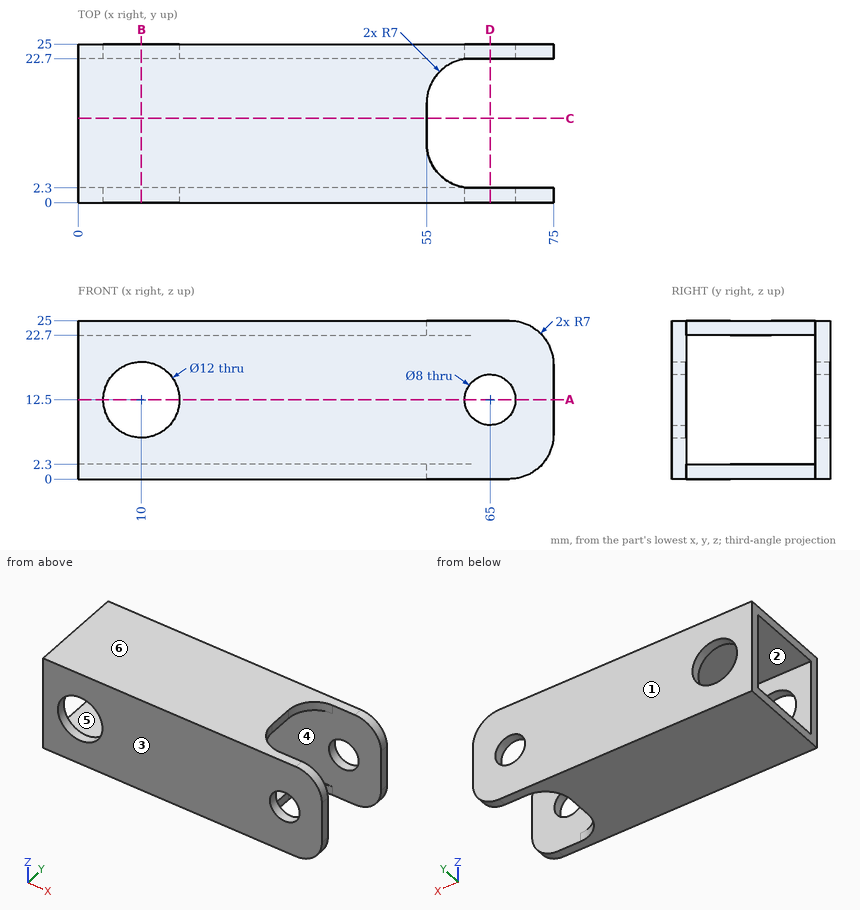
Design review of the part shown in the three views and the two pictorial views. Dimensions are in mm from the part's minimum x, y and z. A direction names the side the tool comes from. Coordinates: 2 decimals unless noted, no trailing zeros. Loops run counter-clockwise (first coordinate to the right, second up) from the corner with the lowest first, then second, coordinate; pieces in that order, holes last.
Q1. We need section B-B on x = 10. State the section outline as (y, z) points, and give its area (3 significant figures).
Reported:
outline: (0, 0) - (25, 0) - (25, 6.5) - (22.7, 6.5) - (22.7, 2.3) - (2.3, 2.3) - (2.3, 6.5) - (0, 6.5) - close; (0, 18.5) - (2.3, 18.5) - (2.3, 22.7) - (22.7, 22.7) - (22.7, 18.5) - (25, 18.5) - (25, 25) - (0, 25) - close
area: 154 mm2
Q2. We need section C-C on y = 13.25. State the section outline as (x, z) points.
Reported:
outline: (0, 0) - (55, 0) - (55, 2.3) - (0, 2.3) - close; (0, 22.7) - (55, 22.7) - (55, 25) - (0, 25) - close
Q3. To check wall thickness, follow line 1 (X direction, y = 23.4, z = 12.5); line 2 (Z direction, x = 10, y = 1.7); line 3 (Z direction, x = 37.5, y = 13). State the ranges of each line that lie inside material, in increasing order.
Reported:
line 1: x = 0 to 4, 16 to 61, 69 to 75
line 2: z = 0 to 6.5, 18.5 to 25
line 3: z = 0 to 2.3, 22.7 to 25
Q4. The part is to be moulded in two halves that separate along Y. For the marked faces 1, 2, 3 and 4, say which applies: +Y half, -Y half, draft (parallel to the pull), parting line (faces both ways), or undercut.
Reported:
face 1: +Y half
face 2: undercut
face 3: -Y half
face 4: undercut
Q5. For pin 1 (10 mm diameter, centred on y = 10, z = 18.5, fed in from +X); pin 2 (1.8 mm diameter, centred on y = 11.5, z = 1, fed in from +X), all flat-tipped, find the tip position at first contact; note any pin that passes through.
Reported:
pin 1: stops at x = 55.3
pin 2: stops at x = 55
Q6. We need section D-D on x = 65. State the section outline as (y, z) points.
Reported:
outline: (0, 0) - (2.3, 0) - (2.3, 8.5) - (0, 8.5) - close; (0, 16.5) - (2.3, 16.5) - (2.3, 25) - (0, 25) - close; (22.7, 0) - (25, 0) - (25, 8.5) - (22.7, 8.5) - close; (22.7, 16.5) - (25, 16.5) - (25, 25) - (22.7, 25) - close
Q7. Tool access review of the marked faces 5 and 6: name each direction out of +Z, -Z, +X, -X, +Y, -Y from which nothing blocks a thin tool from reaching the whole face with its end or side.
Reported:
face 5: +X, -X
face 6: +Z, +X, -X, +Y, -Y
Q8. We need section A-A on z = 12.5. State the section outline as (x, y) points.
Reported:
outline: (0, 0) - (4, 0) - (4, 2.3) - (0, 2.3) - close; (0, 22.7) - (4, 22.7) - (4, 25) - (0, 25) - close; (16, 0) - (61, 0) - (61, 2.3) - (16, 2.3) - close; (16, 22.7) - (61, 22.7) - (61, 25) - (16, 25) - close; (69, 0) - (75, 0) - (75, 2.3) - (69, 2.3) - close; (69, 22.7) - (75, 22.7) - (75, 25) - (69, 25) - close
